Input: part model. Units: mm. Frame: model coordinates. Round coordinates to 2 decimals unless told otherwise and drop trailing zeros. Write each loop counter-clockwise with the first axis right and the second up, starting at its lowest first coordinate (ties: lowest second). Pieces come first, ordered by that corner, then holes. Notation, with made-up numbers: (-30.5, -15.75) -> (22.5, -15.75) arc R30 cw to (22.5, 17.25) -> close; hole circle Ø5 at (14, 39.25). An arc over 180 degrees is marked (long way). Use CSV: the item, a comma, the result in double quotes.
```python
from build123d import *

# Parameters (mm, degrees)
SKETCH_1_W          = 2680
SKETCH_1_H          = 100
EXTRUDE_465_DEPTH   = 8
SKETCH_2_W          = 2680
SKETCH_2_H          = 8
EXTRUDE_1_DEPTH     = 100
CUT_EXTRUDE_1_DEPTH = 100


# Read off the part's stored shape, not the designer's step: 切除-拉伸1
with BuildPart() as part:
    # 草图1 → Extrude 465 (new body)
    with BuildSketch(Plane.XY):
        with Locations((0, 50)):
            Rectangle(SKETCH_1_W, SKETCH_1_H)
    extrude(amount=EXTRUDE_465_DEPTH)

    # 草图2 → 凸台-拉伸1 (add)
    with BuildSketch(Plane.XY.offset(8)):
        with Locations((0, 96)):
            Rectangle(SKETCH_2_W, SKETCH_2_H)
    extrude(amount=EXTRUDE_1_DEPTH)

    # 切除-拉伸1 outline → 切除-拉伸1 (cut)
    with BuildSketch(Plane(origin=(0, 0, 0), x_dir=(1, 0, 0), z_dir=(0, 1, 0))):
        Polygon((1340, -108), (1340, 0), (1070, -108), align=None)
        Polygon((-1340, -108), (-1070, -108), (-1340, 0), align=None)
    extrude(amount=CUT_EXTRUDE_1_DEPTH, mode=Mode.SUBTRACT)


solid = part.part
```
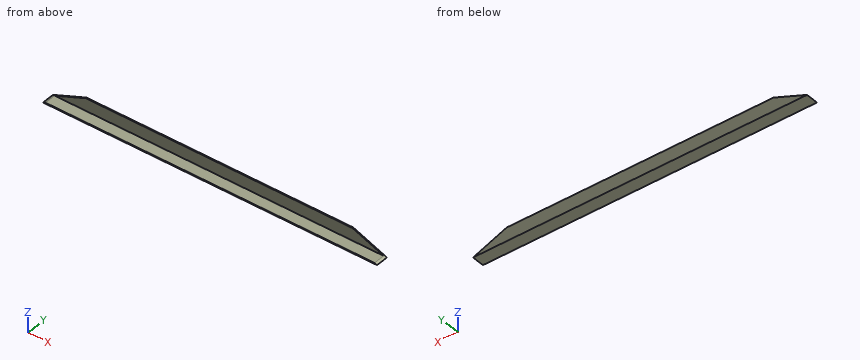
Item 1: Section query A-A on x = 300.5. Return the cut outline in (y, z).
Worked answers:
outline,"(0, 0) -> (100, 0) -> (100, 108) -> (92, 108) -> (92, 8) -> (0, 8) -> close"
Item 2: First-contact query: pin 1 Ø1.5 at (x, z) = (397.5, 19.5) entering from -Y; pin 2 Ø3 at (x, y) = (-763, 40) entering from +Z. Flat tips, straight axial feed; report the tip coordinate or a pass-through.
Worked answers:
pin 1,"stops at y = 92"
pin 2,"stops at z = 8"
Item 3: Line query: line 1 (Z direction, x = -23, y = 69); line 2 (Y direction, x = 696.5, z = 56). Output: solid intervals per line, ascending.
Worked answers:
line 1,"z = 0 to 8"
line 2,"y = 92 to 100"
Item 4: Section query B-B on y = 16.5. Return the cut outline in (x, z), plus the area to 3 significant figures.
Worked answers:
outline,"(-1340, 0) -> (1340, 0) -> (1320, 8) -> (-1320, 8) -> close"
area,"21,300 mm²"
Item 5: Section query C-C on z = 67. Return the cut outline in (x, y).
Worked answers:
outline,"(-1172.5, 92) -> (1172.5, 92) -> (1172.5, 100) -> (-1172.5, 100) -> close"
